Read the model definition and answer for the solid it produces. Units are mm, in the model's axes. Face numbers are marked on the shaded views. A direction names the side the tool comes from. Coordinates: 2 decimals unless noted, no trailing zeros. Loops run counter-clockwise (first coordinate to the right, second up) from the corner with the lowest first, then second, coordinate; pieces in that order, holes last.
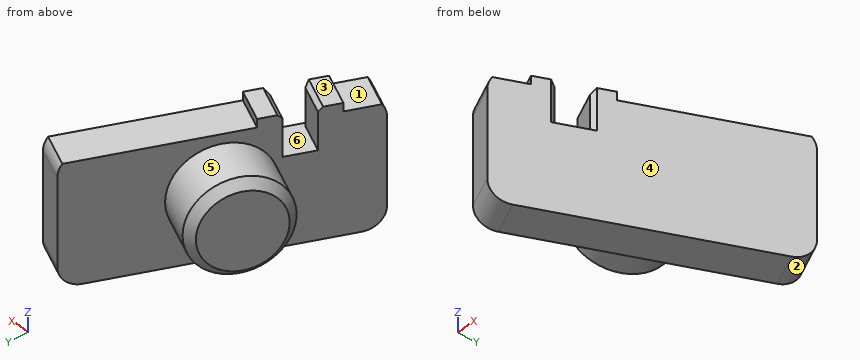
from build123d import *

# Parameters (mm, degrees)
PAD039_DEPTH            = 1.8
SKETCH116_R             = 2.25
PAD040_DEPTH            = 2.6
CHAMFER003_SIZE         = 0.4
SKETCH117_W             = 1.4
SKETCH117_H             = 2
SKETCH117_W_2           = 9.515449
SKETCH117_H_2           = 0.4
SKETCH117_W_3           = 4.064247
POCKET008_DEPTH         = 1.8
CHAMFER004_SIZE         = 0.2
BODY039_PLACEMENT_ANGLE = 23.8


with BuildPart() as part:
    # Sketch115 → Pad039 (new body)
    with BuildSketch(Plane.YZ):
        with BuildLine():
            Line((-6.5, 2.1), (-6.5, -2.1))
            ThreePointArc((-6.5, -2.1), (-6.207107, -2.807107), (-5.5, -3.1))
            Line((-5.5, -3.1), (5.5, -3.1))
            ThreePointArc((5.5, -3.1), (6.207107, -2.807107), (6.5, -2.1))
            Line((6.5, -2.1), (6.5, 2.1))
            ThreePointArc((6.5, 2.1), (6.207107, 2.807107), (5.5, 3.1))
            Line((-5.5, 3.1), (5.5, 3.1))
            ThreePointArc((-5.5, 3.1), (-6.207107, 2.807107), (-6.5, 2.1))
        make_face()
    extrude(amount=PAD039_DEPTH)

    # Sketch116 (on Face9 of Pad039) → Pad040 (join)
    with BuildSketch(Plane(origin=(0, 0, 0), x_dir=(0, 1, 0), z_dir=(-1, 0, 0))):
        Circle(SKETCH116_R)
    extrude(amount=PAD040_DEPTH)

    # Chamfer003
    chamfer003_edges = [part.edges().sort_by_distance(p)[0] for p in [
        (-2.6, -2.25, 0),
    ]]
    chamfer(chamfer003_edges, length=CHAMFER003_SIZE)

    # Sketch117 (on Face13 of Chamfer003) → Pocket008 (cut)
    with BuildSketch(Plane.YZ.offset(1.8)):
        with Locations((-3.08, 2.1)):
            Rectangle(SKETCH117_W, SKETCH117_H)
        with Locations((3.377724, 2.9)):
            Rectangle(SKETCH117_W_2, SKETCH117_H_2)
        with Locations((-6.812123, 2.9)):
            Rectangle(SKETCH117_W_3, SKETCH117_H_2)
    extrude(amount=-POCKET008_DEPTH, mode=Mode.SUBTRACT)

    # Chamfer004
    chamfer004_edges = [part.edges().sort_by_distance(p)[0] for p in [
        (0.9, -2.38, 3.1),
        (0.9, -3.78, 3.1),
        (1.8, -2.38, 2.1),
        (1.8, -3.78, 2.1),
    ]]
    chamfer(chamfer004_edges, length=CHAMFER004_SIZE)


with BuildPart() as part_1:
    # Body039 placement: moved
    add(part.part.moved(Location((-19.5, 50, -6.9))).rotate(Axis((-19.5, 50, -6.9), (0, 0, -1)), BODY039_PLACEMENT_ANGLE))


solid = part_1.part
Q1. Determine the mould class of the marked faces 3, 4, 5 and 6 for opening direction Y: +Y half, -Y half, draft (parallel to the pull), parting line (faces both ways), or undercut.
Findings below:
face 3: draft
face 4: -Y half
face 5: undercut
face 6: undercut
Q2. Straight lines are drawn through the part: probe 1 along Z at (x, y) = (-18.25, 48.75); probe 2 along Z at (x, y) = (-20.5, 47.5); probe 3 along Y at (x, z) = (-21.75, -5.75). For each, find the intervals that lie inside material, in ascending order.
Findings below:
probe 1: z = -10 to -4.2
probe 2: z = -10 to -5.8
probe 3: y = 43.89 to 44.9, 48.88 to 51.34
Q3. A cutting plane is placed at A-A (y = 53.5). Give the vertices of the cut face in (x, z).
Findings below:
outline: (-17.96, -10) - (-15.99, -10) - (-15.99, -4.2) - (-17.96, -4.2) - close
Q4. Flat-ended cylindrical pins translate along their axes: pin 1 Ø1.5 at (x, z) = (-16.5, -5) entering from -Y; pin 2 Ø1.4 at (x, y) = (-17.5, 53) entering from +Z; pin 3 Ø1.5 at (x, z) = (-21.5, -7) entering from +Y. Find the tip coordinate at first contact, or state that the pin passes through.
Findings below:
pin 1: stops at y = 50.64
pin 2: stops at z = -4.2
pin 3: stops at y = 52.89
Q5. A cutting plane is placed at B-B (x = -17.75). Give the vertices of the cut face in (y, z).
Findings below:
outline: (49.51, -10) - (53.97, -10) - (53.97, -4.2) - (49.51, -4.2) - close
Q6. Which of the six approach directions +Z, -Z, +X, -X, +Y, -Y give full straight-line access (tool end or side, diameter ignored) to the marked faces 1 and 2?
Findings below:
face 1: +Z, -X, -Y
face 2: -Z, +X, +Y
